```python
from build123d import *

# Parameters (mm, degrees)
SKETCH1_R           = 5.25
BOSS_EXTRUDE1_DEPTH = 50
SKETCH2_R           = 4.75
CUT_EXTRUDE1_DEPTH  = 50
FILLET1_R           = 1


with BuildPart() as part:
    # Sketch1 → Boss-Extrude1 (new body)
    with BuildSketch(Plane(origin=(0, 0, 0), x_dir=(1, 0, 0), z_dir=(0, 1, 0))):
        with Locations(Location((0, 0, 0), (0, 0, 270))):
            Circle(SKETCH1_R)
    extrude(amount=BOSS_EXTRUDE1_DEPTH)

    # Sketch2 → Cut-Extrude1 (cut)
    with BuildSketch(Plane(origin=(0, 50, 0), x_dir=(1, 0, 0), z_dir=(0, 1, 0))):
        with Locations(Location((0, 0, 0), (0, 0, 270))):
            Circle(SKETCH2_R)
    extrude(amount=-CUT_EXTRUDE1_DEPTH, mode=Mode.SUBTRACT)

    # Fillet1
    # the kernel refuses this fillet: 1 mm, written as the material it takes off along each edge
    with BuildSketch(Plane(origin=(0, 0, 0), x_dir=(0, 0, 1), z_dir=(-1, 0, 0))) as fillet1_piece_1:
        with BuildLine():
            CenterArc((4.25, 0.866025404), FILLET1_R, 300, 60)
            Line((4.75, 0), (4.76, -0.017320508))
            ThreePointArc((4.76, -0.017320508), (5, -0.02), (5.25, -0.02))
            Line((5.25, -0.02), (5.27, 0))
            Line((5.27, 0), (5.27, 0.866025404))
            Line((5.27, 0.866025404), (5.25, 0.866025404))
        make_face()
    revolve(axis=Axis((0, 0, 0), (0, 1, 0)), mode=Mode.SUBTRACT)
    with BuildSketch(Plane(origin=(0, 50, 0), x_dir=(0, 0, 1), z_dir=(-1, 0, 0))) as fillet1_piece_2:
        with BuildLine():
            CenterArc((4.25, -0.866025404), FILLET1_R, 0, 60)
            Line((4.75, 0), (4.76, 0.017320508))
            ThreePointArc((4.76, 0.017320508), (5, 0.02), (5.25, 0.02))
            Line((5.25, 0.02), (5.27, 0))
            Line((5.27, 0), (5.27, -0.866025404))
            Line((5.27, -0.866025404), (5.25, -0.866025404))
        make_face()
    revolve(axis=Axis((0, 50, 0), (0, 1, 0)), mode=Mode.SUBTRACT)


solid = part.part
```
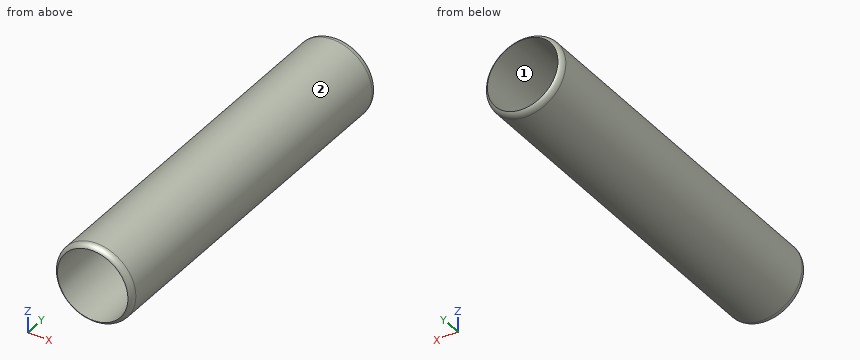
Can you work these out from the model? Positions are in its coordinate system, mm. Face numbers are marked on the shaded views. Give positions to 0.01 mm unless a question says otherwise; leave off trailing zeros. Loops run counter-clockwise (first coordinate to the right, second up) from the corner with the lowest first, then second, coordinate; pieces in that order, holes last. Notation, with made-up numbers: M -9.75,24 L 31.25,24 A20 ccw 31.25,39 Z; hole C 39,58.25 d2. An arc over 180 degrees is marked long. One line per question, with ' | ' between items. Start each with the question number.
Q1. If we section it at A-A (x = 0): Please give me the cut outline in (y, z).
Q2. If we mould it in two halves opening along Z, with no side actions, what happens to the marked faces 1 and 2? For each: +Z half, -Z half, draft (parallel to the pull), parting line (faces both ways), or undercut.
Q3. If we section it at C-C (y = 37): Please give me the cut outline in (x, z).
Q4. If we section it at B-B (z = 0): Please give me the cut outline in (x, y).
Q5. For pin 1 Ø4 at (x, z) = (-1, -1.5) entering from +Y; pin 2 Ø3 at (x, y) = (-4, 8) entering from +Z, each with a flat end and sliding along its axis, tell me the tip position at first contact or that it passes through.
Q6. If I drill on line 1 (X direction, y = 35.5, z = 0); line 2 (X direction, y = 22, z = 3.5); line 3 (Z direction, x = 3, y = 41.5), over which ranges is the centre line in solid material (lowest first)? Write a range as from..to.
Computed:
1) outline: M 0,-4.75 A1 ccw 0.87,-5.25 L 49.13,-5.25 A1 ccw 50,-4.75 Z; M 0,4.75 L 50,4.75 A1 ccw 49.13,5.25 L 0.87,5.25 A1 ccw Z
2) face 1: undercut | face 2: parting line
3) outline: C 0,0 d10.5; hole C 0,0 d9.5
4) outline: M -5.25,0.87 A1 ccw -4.75,0 L -4.75,50 A1 ccw -5.25,49.13 Z; M 4.75,0 A1 ccw 5.25,0.87 L 5.25,49.13 A1 ccw 4.75,50 Z
5) pin 1: passes through | pin 2: stops at z = 4.62
6) line 1: x = -5.25..-4.75, 4.75..5.25 | line 2: x = -3.91..-3.21, 3.21..3.91 | line 3: z = -4.31..-3.68, 3.68..4.31
